from build123d import *

# Parameters (mm, degrees)
ESQUISSE2_W             = 8
ESQUISSE2_H             = 20
ESQUISSE2_R             = 2.25
BOSS_EXTRU_1_DEPTH      = 10
BOSS_EXTRU_1_2_DEPTH    = 10
BOSS_EXTRU_2_DEPTH      = 3
BOSS_EXTRU_5_DEPTH      = 93
ENL_V_MAT_EXTRU_1_REACH = 18
ESQUISSE8_W             = 8
ESQUISSE8_H             = 30
ESQUISSE9_W             = 80.2
ESQUISSE9_H             = 8.2
ENL_V_MAT_EXTRU_2_DEPTH = 2
ESQUISSE10_W            = 8
ESQUISSE10_H            = 14
ESQUISSE10_R            = 1.65
BOSS_EXTRU_6_DEPTH      = 5


with BuildPart() as part:
    # Esquisse2 → Boss.-Extru.1 (new body)
    with BuildSketch(Plane(origin=(0, 0, 0), x_dir=(0, 0, -1), z_dir=(1, 0, 0))):
        with Locations((-24, 0)):
            Rectangle(ESQUISSE2_W, ESQUISSE2_H)
        with Locations((-24, 5)):
            Circle(ESQUISSE2_R, mode=Mode.SUBTRACT)
        with Locations((-24, -5)):
            Circle(ESQUISSE2_R, mode=Mode.SUBTRACT)
    extrude(amount=BOSS_EXTRU_1_DEPTH)



with BuildPart() as body_2:
    # Esquisse2 → Boss.-Extru.1 2 (new body)
    with BuildSketch(Plane(origin=(0, 0, 0), x_dir=(0, 0, -1), z_dir=(1, 0, 0))):
        with Locations((24, 0)):
            Rectangle(ESQUISSE2_W, ESQUISSE2_H)
        with Locations((24, 5)):
            Circle(ESQUISSE2_R, mode=Mode.SUBTRACT)
        with Locations((24, -5)):
            Circle(ESQUISSE2_R, mode=Mode.SUBTRACT)
    extrude(amount=BOSS_EXTRU_1_2_DEPTH)


with BuildPart() as part_1:
    add(part.part)

    add(body_2.part)  # Boss.-Extru.2 merges body 2
    # Esquisse3 → Boss.-Extru.2 (add)
    with BuildSketch(Plane.XZ.offset(10)):
        Polygon((-60, 28), (-60, -72), (33, -72), (33, -28), (10, -28), (10, 28), align=None)
    extrude(amount=BOSS_EXTRU_2_DEPTH)

    # Esquisse7 → Boss.-Extru.5 (add)
    with BuildSketch(Plane(origin=(33, 0, 0), x_dir=(0, 0, -1), z_dir=(1, 0, 0))):
        Polygon((72, -10), (81, -10), (81, -26), (74, -26), (74, -13), (72, -13), align=None)
    extrude(amount=-BOSS_EXTRU_5_DEPTH)

    # Esquisse8 → Enlèv. mat.-Extru.1 (cut, up to next)
    with BuildSketch(Plane(origin=(0, -10, 0), x_dir=(1, 0, 0), z_dir=(0, 1, 0)), mode=Mode.PRIVATE) as enl_v_mat_extru_1_sk1:
        with Locations((-56, -13)):
            Rectangle(ESQUISSE8_W, ESQUISSE8_H)
    enl_v_mat_extru_1_tool1 = extrude(enl_v_mat_extru_1_sk1.sketch, amount=-ENL_V_MAT_EXTRU_1_REACH, mode=Mode.PRIVATE) & part_1.part
    add(enl_v_mat_extru_1_tool1.solids().sort_by_distance((-56, -10, 13))[0], mode=Mode.SUBTRACT)

    # Esquisse9 → Enlèv. mat.-Extru.2 (cut)
    with BuildSketch(Plane.XY.offset(-74)):
        with Locations((-13.5, -19.5)):
            Rectangle(ESQUISSE9_W, ESQUISSE9_H)
    extrude(amount=-ENL_V_MAT_EXTRU_2_DEPTH, mode=Mode.SUBTRACT)

    # Esquisse10 → Boss.-Extru.6 (add)
    with BuildSketch(Plane.ZY.offset(52)):
        with Locations((10, -3)):
            Rectangle(ESQUISSE10_W, ESQUISSE10_H)
        with Locations((10, 0)):
            Circle(ESQUISSE10_R, mode=Mode.SUBTRACT)
    extrude(amount=-BOSS_EXTRU_6_DEPTH)


solid = part_1.part
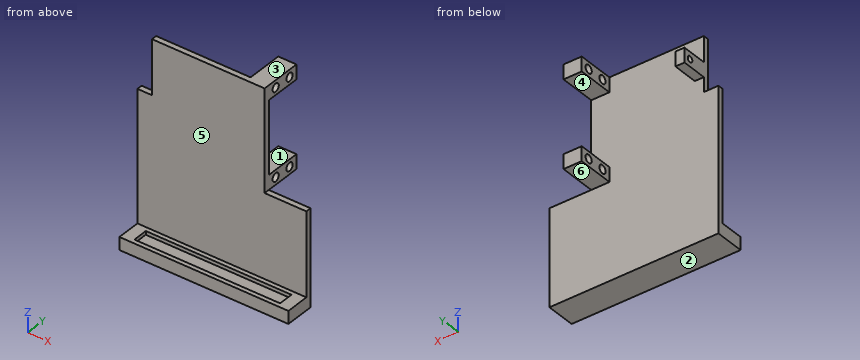
Could you check a few things on this model? Use its own coordinates, in mm. Face numbers are marked on the shaded views. A direction names the side the tool comes from. Round coordinates to 2 decimals unless told otherwise and drop trailing zeros. Write each loop counter-clockwise with the first axis right and the second up, starting at its lowest first coordinate (ties: lowest second). Pieces come first, ordered by that corner, then holes. Notation, with made-up numbers: (37.5, 47) -> (74.5, 47) arc R6 cw to (74.5, 54) -> close; hole circle Ø1 at (3, 7.25). An arc over 180 degrees is marked (long way). Use a Markdown table: item, result.
1. If we section it at D-D (x = -2): List the corners of the cut face in (y, z) for me.
Answer key:
| item | result |
|---|---|
| outline | (-26, -81) -> (-10, -81) -> (-10, 28) -> (-13, 28) -> (-13, -74) -> (-15.4, -74) -> (-15.4, -76) -> (-23.6, -76) -> (-23.6, -74) -> (-26, -74) -> close |
2. Please list where these lines run through material, in increasing order: probe 1 along Y at (x, z) = (2, 24); probe 2 along Z at (x, y) = (-51.5, -19.5); probe 3 along X at (y, z) = (-10.5, 16.5).
Answer key:
| item | result |
|---|---|
| probe 1 | y = -13 to -7.25, -2.75 to 2.75, 7.25 to 10 |
| probe 2 | z = -81 to -76 |
| probe 3 | x = -52 to 10 |
3. We'd pull the mould along Z, two halves only. Please class the marked faces 1, 2, 3 and 4: +Z half, -Z half, draft (parallel to the pull), parting line (faces both ways), or undercut.
Answer key:
| item | result |
|---|---|
| face 1 | undercut |
| face 2 | -Z half |
| face 3 | +Z half |
| face 4 | undercut |
4. For pin 1 Ø12 at (x, y) = (-48.5, 5.5) entering from -Z; pin 2 Ø1.5 at (x, z) = (-30.5, -21) entering from -Y; pin 3 Ø6 at (y, z) = (5, 24) entering from +X; pin 4 Ø3.5 at (y, z) = (5, -24) entering from -X, each with a flat end and sliding along its axis, tell me the tip position at first contact or that it passes through.
Answer key:
| item | result |
|---|---|
| pin 1 | stops at z = 6 |
| pin 2 | stops at y = -13 |
| pin 3 | stops at x = 10 |
| pin 4 | passes through |
5. If we section it at C-C (z = 10): List the corners of the cut face in (x, y) for me.
Answer key:
| item | result |
|---|---|
| outline | (-52, -13) -> (10, -13) -> (10, -10) -> (-47, -10) -> (-47, -1.65) -> (-52, -1.65) -> close; (-52, 1.65) -> (-47, 1.65) -> (-47, 4) -> (-52, 4) -> close |
6. If we section it at B-B (y = 0): List the corners of the cut face in (x, z) for me.
Answer key:
| item | result |
|---|---|
| outline | (-52, 6) -> (-47, 6) -> (-47, 8.35) -> (-52, 8.35) -> close; (-52, 11.65) -> (-47, 11.65) -> (-47, 14) -> (-52, 14) -> close; (0, -28) -> (10, -28) -> (10, -20) -> (0, -20) -> close; (0, 20) -> (10, 20) -> (10, 28) -> (0, 28) -> close |
7. Which directions (+Z, -Z, +X, -X, +Y, -Y) give clear straight access to the entire face, cutting with the end or side of a thin tool? Please do the marked faces 5 and 6.
Answer key:
| item | result |
|---|---|
| face 5 | +Z, +X, -X, -Y |
| face 6 | -Z, +X, -X, +Y |
8. If we section it at A-A (z = -24): List the corners of the cut face in (x, y) for me.
Answer key:
| item | result |
|---|---|
| outline | (-60, -13) -> (10, -13) -> (10, -7.25) -> (0, -7.25) -> (0, -10) -> (-60, -10) -> close; (0, -2.75) -> (10, -2.75) -> (10, 2.75) -> (0, 2.75) -> close; (0, 7.25) -> (10, 7.25) -> (10, 10) -> (0, 10) -> close |
